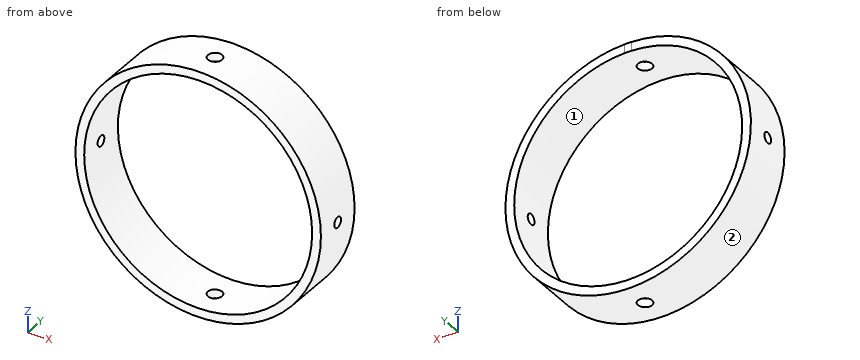
```python
from build123d import *

# Parameters (mm, degrees)
SKETCH1_R                       = 44.45
SKETCH1_R_2                     = 41.275
BOSS_EXTRUDE1_DEPTH             = 19.05
SKETCH5_W                       = 2.5527
SKETCH5_H                       = 76.2
TAP_DRILL_FOR_1_4_20_TAP2_D     = 5.1054
TAP_DRILL_FOR_1_4_20_TAP2_DEPTH = 76.2
SKETCH10_R                      = 1.905
CUT_EXTRUDE3_DEPTH              = 77.2000001
CUT_EXTRUDE3_DEPTH_BACK         = 13.7000001
TIGWELD_W                       = 2.542332396
TIGWELD_H                       = 3.176399095
BOSS_EXTRUDE2_DEPTH             = 0.0254


with BuildPart() as part:
    # Sketch1 → Boss-Extrude1 (new body)
    with BuildSketch(Plane(origin=(0, 0, 0), x_dir=(1, 0, 0), z_dir=(0, 1, 0))):
        Circle(SKETCH1_R)
        Circle(SKETCH1_R_2, mode=Mode.SUBTRACT)
    extrude(amount=BOSS_EXTRUDE1_DEPTH)

    # Sketch5 → Tap Drill for 1/4-20 Tap1 (revolve, cut)
    with BuildSketch(Plane(origin=(0, 9.525, 31.75), x_dir=(0, -1, 0), z_dir=(1, 0, 0))):
        with Locations((1.27635, 38.1)):
            Rectangle(SKETCH5_W, SKETCH5_H)
    revolve(axis=Axis((0, 9.525, 38.1), (0, 0, -1)), mode=Mode.SUBTRACT)

    # Tap Drill for 1/4-20 Tap2
    with Locations(Plane(origin=(0, 0, -31.75), x_dir=(1, 0, 0), z_dir=(0, 0, -1))):
        with Locations((0, -9.525)):
            Hole(TAP_DRILL_FOR_1_4_20_TAP2_D / 2, depth=TAP_DRILL_FOR_1_4_20_TAP2_DEPTH)

    # Sketch10 → Cut-Extrude3 (cut, two sides)
    with BuildSketch(Plane(origin=(-31.75, 0, 0), x_dir=(0, 0, -1), z_dir=(1, 0, 0))) as cut_extrude3_sk:
        with Locations((0, 9.487883811)):
            Circle(SKETCH10_R)
    extrude(amount=CUT_EXTRUDE3_DEPTH, mode=Mode.SUBTRACT)
    extrude(cut_extrude3_sk.sketch, amount=-CUT_EXTRUDE3_DEPTH_BACK, mode=Mode.SUBTRACT)

    # TigWeld → Boss-Extrude2 (add)
    with BuildSketch(Plane(origin=(0, 19.05, 0), x_dir=(1, 0, 0), z_dir=(0, 1, 0))):
        with Locations((0, -42.843620543)):
            Rectangle(TIGWELD_W, TIGWELD_H)
    extrude(amount=BOSS_EXTRUDE2_DEPTH)


solid = part.part
```
The listing builds one solid part. Answer for the finished solid, in the listing's coordinates (mm). Face numbers are marked on the shaded views. Round coordinates to 2 decimals unless told otherwise and drop trailing zeros. Loops run counter-clockwise (first coordinate to the right, second up) from the corner with the lowest first, then second, coordinate; pieces in that order, holes last.
1) A cutting plane is placed at A-A on x = 0. Determine the outline of the cut face in (y, z) (3 decimals), plus the area to 3 significant figures.
Outcome:
outline: (0, -44.45) - (6.972, -44.45) - (6.972, -41.275) - (0, -41.275) - close; (0, 41.275) - (6.972, 41.275) - (6.972, 44.45) - (0, 44.45) - close; (12.078, -44.45) - (19.05, -44.45) - (19.05, -41.275) - (12.078, -41.275) - close; (12.078, 41.275) - (19.05, 41.275) - (19.05, 41.255) - (19.075, 41.255) - (19.075, 44.432) - (19.05, 44.432) - (19.05, 44.45) - (12.078, 44.45) - close
area: 88.6 mm2
2) A cutting plane is placed at B-B on z = 6. Determine the outline of the cut face in (x, y), plus the area to 3 significant figures.
Outcome:
outline: (-44.04, 0) - (-40.84, 0) - (-40.84, 19.05) - (-44.04, 19.05) - close; (40.84, 0) - (44.04, 0) - (44.04, 19.05) - (40.84, 19.05) - close
area: 122 mm2
3) Consider line 1 (Y direction, x = -42.15, z = 0); line 2 (Y direction, x = 0, z = -42.6); line 3 (X direction, y = 12.25, z = 0) (3 decimals). Determine where each line is inside the solid, lowest interval first.
Outcome:
line 1: y = 0 to 7.58, 11.39 to 19.05
line 2: y = 0 to 6.97, 12.08 to 19.05
line 3: x = -44.45 to -41.275, 41.275 to 44.45
4) A cutting plane is placed at C-C on x = -20.5. Determine the outline of the cut face in (y, z), plus the area to 3 significant figures.
Outcome:
outline: (0, -39.44) - (19.05, -39.44) - (19.05, -35.82) - (0, -35.82) - close; (0, 35.82) - (19.05, 35.82) - (19.05, 39.44) - (0, 39.44) - close
area: 138 mm2
5) A cutting plane is placed at D-D on y = 17.75. Determine the outline of the cut face in (x, z) (3 decimals).
Outcome:
outline: circle Ø88.9 at (0, 0); hole circle Ø82.55 at (0, 0)
6) For a pull along X with two mould halves and no side action, classify the marked faces 1 and 2 as released by +X, released by -X, zero draft, split by the parting line, or undercut.
Outcome:
face 1: undercut
face 2: split by the parting line
7) Given P1, Ø12, axis at x = -20.5, z = -34.5, coming from the +Y side; P2, Ø3, axis at x = 0, y = 9.525, coming from the +Z side; P3, Ø2, axis at y = 10, z = -12.5, coming from the +X side; P4, Ø8, axis at y = 12.5, z = 30, coming from the +X side, each flat-ended and moving along its own axis, determine where each tip first touches the part or whether it passes through.
Outcome:
P1: stops at y = 19.05
P2: passes through
P3: stops at x = 42.94
P4: stops at x = 36.05
